from build123d import *

# Parameters (mm, degrees)
SKETCH_1_R      = 1.65
SKETCH_1_R_2    = 1
EXTRUDE_1_DEPTH = 2
FILLET_1_R      = 1


with BuildPart() as part:
    # Эскиз1 → Бобышка-Вытянуть1 (new body)
    with BuildSketch(Plane(origin=(0, 0, 0), x_dir=(1, 0, 0), z_dir=(0, 1, 0))):
        with BuildLine():
            Line((0, 10), (90, 10))
            Line((90, 10), (90, -10))
            Line((90, -10), (0, -10))
            ThreePointArc((0, -10), (-10, 0), (0, 10))
        make_face()
        with Locations(Location((30, 0, 0), (0, 0, 270))):
            Circle(SKETCH_1_R, mode=Mode.SUBTRACT)
        with Locations(Location((0, 0, 0), (0, 0, 270))):
            Circle(SKETCH_1_R, mode=Mode.SUBTRACT)
        with Locations(Location((15, 0, 0), (0, 0, 270))):
            Circle(SKETCH_1_R, mode=Mode.SUBTRACT)
        with Locations(Location((87.5, 7.5, 0), (0, 0, 270))):
            Circle(SKETCH_1_R_2, mode=Mode.SUBTRACT)
        with Locations(Location((72.5, 7.5, 0), (0, 0, 270))):
            Circle(SKETCH_1_R_2, mode=Mode.SUBTRACT)
        with Locations(Location((87.5, -7.5, 0), (0, 0, 270))):
            Circle(SKETCH_1_R_2, mode=Mode.SUBTRACT)
        with Locations(Location((72.5, -7.5, 0), (0, 0, 270))):
            Circle(SKETCH_1_R_2, mode=Mode.SUBTRACT)
    extrude(amount=EXTRUDE_1_DEPTH)

    # Скругление1
    fillet_1_edges = [part.edges().sort_by_distance(p)[0] for p in [
        (90, 1, -10),
        (90, 1, 10),
    ]]
    fillet(fillet_1_edges, radius=FILLET_1_R)


solid = part.part
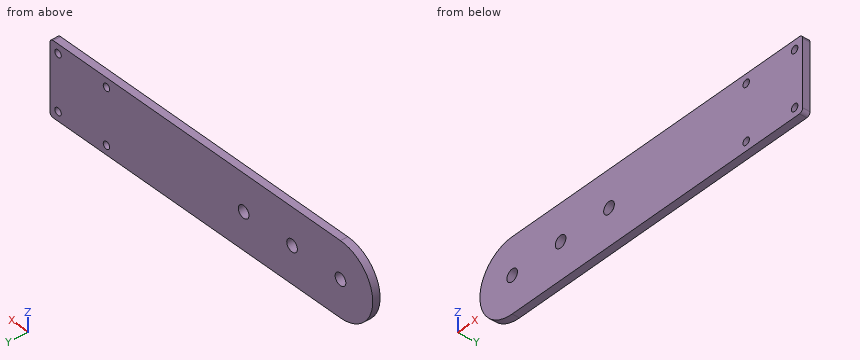
Design review of the part built by this model. Coordinates are the model's own, in mm. Coordinates: 2 decimals unless noted, no trailing zeros. Loops run counter-clockwise (first coordinate to the right, second up) from the corner with the lowest first, then second, coordinate; pieces in that order, holes last. Notation, with made-up numbers: (-0.5, 47.5) -> (50.5, 47.5) arc R17 cw to (50.5, 52.5) -> close; hole circle Ø1 at (59.25, 53). An arc over 180 degrees is marked (long way). Use a Markdown table: item, result. Add a question column.
Item 1: We need section B-B, the plane x = 15. Write out the cut boundary in (y, z), and give its area (3 significant figures).
Item 2: Wall thickness on L1, parallel to X at y = 0.7, z = 0.25; L2, parallel to Z at x = 87.5, y = 0.5; L3, parallel to X at y = 1.1, z = -7.5: over which ranges is each line inside the solid? List them lowest first. Write a range as from..to.
Item 3: We need section D-D, the plane y = 0.5. Write out the cut boundary in (x, z), and give its area (3 significant figures).
Item 4: We need section A-A, the plane z = 0. Write out the cut boundary in (x, y), and give its area (3 significant figures).
Item 5: We need section C-C, the plane x = 72.5. Write out the cut boundary in (y, z).
Item 6: Clearance check with flat-ended pins moving along their axes: P1, Ø1.6, axis at x = 72.5, z = 7.5, coming from the +Y side; P2, Ø1, axis at y = 1, z = 2, coming from the -X side. State where each tip first meets the part, or that it passes through.
Numbers:
| question | item | result |
|---|---|---|
| 1 | outline | (0, -10) -> (2, -10) -> (2, -1.65) -> (0, -1.65) -> close; (0, 1.65) -> (2, 1.65) -> (2, 10) -> (0, 10) -> close |
| 1 | area | 33.4 mm^2 |
| 2 | L1 | x = -10..-1.63, 1.63..13.37, 16.63..28.37, 31.63..90 |
| 2 | L2 | z = -10..-8.5, -6.5..6.5, 8.5..10 |
| 2 | L3 | x = -6.61..71.5, 73.5..86.5, 88.5..90 |
| 3 | outline | (0, -10) -> (89, -10) arc R1 ccw to (90, -9) -> (90, 9) arc R1 ccw to (89, 10) -> (0, 10) arc R10 ccw to start; hole circle Ø3.3 at (0, 0); hole circle Ø3.3 at (15, 0); hole circle Ø3.3 at (30, 0); hole circle Ø2 at (72.5, -7.5); hole circle Ø2 at (72.5, 7.5); hole circle Ø2 at (87.5, -7.5); hole circle Ø2 at (87.5, 7.5) |
| 3 | area | 1,920 mm^2 |
| 4 | outline | (-10, 0) -> (-1.65, 0) -> (-1.65, 2) -> (-10, 2) -> close; (1.65, 0) -> (13.35, 0) -> (13.35, 2) -> (1.65, 2) -> close; (16.65, 0) -> (28.35, 0) -> (28.35, 2) -> (16.65, 2) -> close; (31.65, 0) -> (90, 0) -> (90, 2) -> (31.65, 2) -> close |
| 4 | area | 180 mm^2 |
| 5 | outline | (0, -10) -> (2, -10) -> (2, -8.5) -> (0, -8.5) -> close; (0, -6.5) -> (2, -6.5) -> (2, 6.5) -> (0, 6.5) -> close; (0, 8.5) -> (2, 8.5) -> (2, 10) -> (0, 10) -> close |
| 6 | P1 | passes through |
| 6 | P2 | stops at x = -9.89 |
